Part model, mm, in its own coordinate system. Face numbers are marked on the shaded views. A direction names the side the tool comes from. Round coordinates to 2 decimals unless told otherwise and drop trailing zeros. Write each loop counter-clockwise with the first axis right and the second up, starting at its lowest first coordinate (ties: lowest second). Pieces come first, ordered by that corner, then holes.
```python
from build123d import *

# Parameters (mm, degrees)
SKETCH1_R                                    = 30
SKETCH1_R_2                                  = 20
BOSS_EXTRUDE1_DEPTH                          = 40
SKETCH2_W                                    = 2
SKETCH2_H                                    = 30
CUT_EXTRUDE1_DEPTH                           = 59.309518948
BOSS_EXTRUDE2_START                          = -40
BOSS_EXTRUDE2_DEPTH                          = 40
CBORE_FOR_M4_HEX_SOCKET_HEAD_CAP_SCR_2_COUNT = 2
CBORE_FOR_M4_HEX_SOCKET_HEAD_CAP_SCR_2_PITCH = 12
CBORE_FOR_M4_HEX_SOCKET_HEAD_CAP_SCR_3_COUNT = 2
CBORE_FOR_M4_HEX_SOCKET_HEAD_CAP_SCR_3_PITCH = 24
SKETCH6_R                                    = 3.75
CUT_EXTRUDE2_DEPTH                           = 66.946948375
F_5_4_5_4_DIAMETER_HOLE1_D                   = 4.2
SKETCH10_R                                   = 3
CUT_EXTRUDE3_DEPTH                           = 11
BOSS_EXTRUDE4_DEPTH                          = 20
BOSS_EXTRUDE4_DEPTH_BACK                     = 20
SKETCH13_R                                   = 17.5
SKETCH13_R_2                                 = 10
FILLET1_R                                    = 15


with BuildPart() as part:
    # Sketch1 → Boss-Extrude1 (new body)
    with BuildSketch(Plane(origin=(0, 0, 0), x_dir=(1, 0, 0), z_dir=(0, 1, 0))):
        with Locations(Location((0, 0, 0), (0, 0, 270))):
            Circle(SKETCH1_R)
        with Locations(Location((0, 0, 0), (0, 0, 270))):
            Circle(SKETCH1_R_2, mode=Mode.SUBTRACT)
    extrude(amount=BOSS_EXTRUDE1_DEPTH)

    # Sketch2 → Cut-Extrude1 (cut, through all)
    with BuildSketch(Plane(origin=(0, 40, 0), x_dir=(1, 0, 0), z_dir=(0, 1, 0))):
        with Locations((0, -15)):
            Rectangle(SKETCH2_W, SKETCH2_H)
    extrude(amount=-CUT_EXTRUDE1_DEPTH, mode=Mode.SUBTRACT)

    # Sketch3 → Boss-Extrude2 (add)
    with BuildSketch(Plane(origin=(0, 40, 0), x_dir=(1, 0, 0), z_dir=(0, 1, 0)).offset(BOSS_EXTRUDE2_START)):
        with BuildLine():
            Line((-1, -29.983328701), (-13, -29.983328701))
            Line((-13, -29.983328701), (-13, -27.037011669))
            ThreePointArc((-13, -27.037011669), (-7.153334608, -29.134683866), (-1, -29.983328701))
        make_face()
    extrude(amount=BOSS_EXTRUDE2_DEPTH)

    # Sketch5 → CBORE for M4 Hex Socket Head Cap Screw1 (revolve, cut)
    with BuildSketch(Plane(origin=(-13, 32, 24.979156528), x_dir=(0, 0, 1), z_dir=(0, 1, 0))):
        Polygon((0, 0), (0, 13.351936393), (2.25, 12), (2.25, 4), (3.75, 4), (3.75, 0), align=None)
    cbore_for_m4_hex_socket_head_cap_screw1 = revolve(axis=Axis((-19.35, 32, 24.979156528), (1, 0, 0)), mode=Mode.SUBTRACT)

    # CBORE for M4 Hex Socket Head Cap Scr 2: CBORE for M4 Hex Socket Head Cap Screw1 ×2
    with Locations(*[(0, -i * CBORE_FOR_M4_HEX_SOCKET_HEAD_CAP_SCR_2_PITCH, 0) for i in range(1, CBORE_FOR_M4_HEX_SOCKET_HEAD_CAP_SCR_2_COUNT)]):
        add(cbore_for_m4_hex_socket_head_cap_screw1, mode=Mode.SUBTRACT)

    # CBORE for M4 Hex Socket Head Cap Scr 3: CBORE for M4 Hex Socket Head Cap Screw1 ×2
    with Locations(*[(0, -i * CBORE_FOR_M4_HEX_SOCKET_HEAD_CAP_SCR_3_PITCH, 0) for i in range(1, CBORE_FOR_M4_HEX_SOCKET_HEAD_CAP_SCR_3_COUNT)]):
        add(cbore_for_m4_hex_socket_head_cap_screw1, mode=Mode.SUBTRACT)

    # Sketch6 → Cut-Extrude2 (cut, through all)
    with BuildSketch(Plane.ZY.offset(13)):
        with Locations((24.979156528, 32)):
            Circle(SKETCH6_R)
        with Locations((24.979156528, 20)):
            Circle(SKETCH6_R)
        with Locations((24.979156528, 8)):
            Circle(SKETCH6_R)
    extrude(amount=CUT_EXTRUDE2_DEPTH, mode=Mode.SUBTRACT)

    # Ø5.4 (5.4) Diameter Hole1 (through all)
    with Locations(Plane.ZY.offset(-1)):
        with Locations((24.979156528, 8), (24.979156528, 20), (24.979156528, 32)):
            Hole(F_5_4_5_4_DIAMETER_HOLE1_D / 2)

    # Sketch10 → Cut-Extrude3 (cut)
    with BuildSketch(Plane.ZY.offset(-22)):
        with Locations((24.979156528, 8)):
            Circle(SKETCH10_R)
        with Locations((24.979156528, 32)):
            Circle(SKETCH10_R)
        with Locations((24.979156528, 20)):
            Circle(SKETCH10_R)
    extrude(amount=CUT_EXTRUDE3_DEPTH, mode=Mode.SUBTRACT)

    # Sketch13 → Boss-Extrude4 (add, two sides: drawn at the far end of the back side and taken through both)
    # profile 1 of 3: a face of its own
    with BuildSketch(Plane(origin=(0, 0, 0), x_dir=(0, 0, -1), z_dir=(1, 0, 0)).offset(-BOSS_EXTRUDE4_DEPTH_BACK)):
        with BuildLine():
            ThreePointArc((28.5, 20), (33.625631329, 32.374368671), (46, 37.5))
            Line((46, 37.5), (30, 37.5))
            Line((30, 37.5), (28.5, 37.5))
            Line((28.5, 37.5), (28.5, 20))
        make_face()
    # profile 2 of 3: a face of its own
    with BuildSketch(Plane(origin=(0, 0, 0), x_dir=(0, 0, -1), z_dir=(1, 0, 0)).offset(-BOSS_EXTRUDE4_DEPTH_BACK)):
        with BuildLine():
            ThreePointArc((46, 2.5), (33.625631329, 7.625631329), (28.5, 20))
            Line((28.5, 20), (28.5, 2.5))
            Line((28.5, 2.5), (30, 2.5))
            Line((30, 2.5), (46, 2.5))
        make_face()
    # profile 3 of 3: a face of its own
    with BuildSketch(Plane(origin=(0, 0, 0), x_dir=(0, 0, -1), z_dir=(1, 0, 0)).offset(-BOSS_EXTRUDE4_DEPTH_BACK)):
        with Locations((46, 20)):
            Circle(SKETCH13_R)
        with Locations((46, 20)):
            Circle(SKETCH13_R_2, mode=Mode.SUBTRACT)
    extrude(amount=BOSS_EXTRUDE4_DEPTH + BOSS_EXTRUDE4_DEPTH_BACK)

    # Fillet1
    # the kernel refuses this fillet: 15 mm, written as the material it adds along each edge
    with BuildSketch(Plane(origin=(9.367496998, 37.5, -28.5), x_dir=(0.8228917781054501, 0, 0.5681981357998729), z_dir=(0, -1, 0))) as fillet1_piece_1:
        with BuildLine():
            CenterArc((21.213026524, -14.387505004), FILLET1_R, 106.429799285, 39.762375137)
            Line((8.749399301, -6.041368385), (0, 0))
            ThreePointArc((0, 0), (8.48521061, -1.224989993), (16.970421219, 0))
        make_face()
    extrude(amount=35)
    with BuildSketch(Plane(origin=(-9.367496998, 37.5, -28.5), x_dir=(-0.8228917781054502, 0, 0.5681981357998726), z_dir=(0, -1, 0))) as fillet1_piece_2:
        with BuildLine():
            CenterArc((21.213026524, 14.387505004), FILLET1_R, 213.807825578, 39.762375137)
            Line((8.749399301, 6.041368385), (0, 0))
            ThreePointArc((0, 0), (8.48521061, 1.224989993), (16.970421219, 0))
        make_face()
    extrude(amount=35)


solid = part.part
```
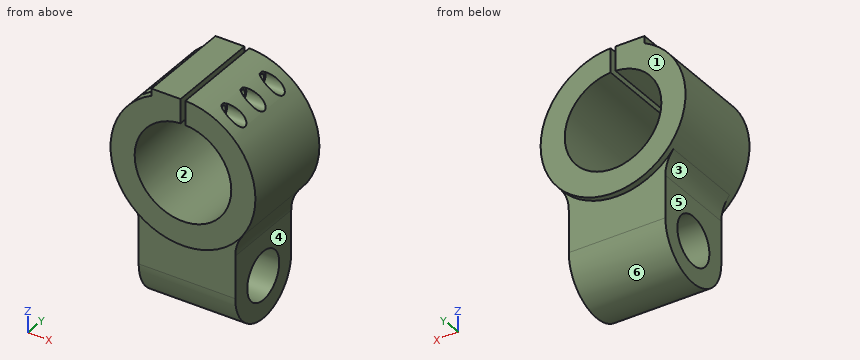
Q1. Cut at D-D on y = 26.5. Write the cut outline in (x, z), plus the area to 3 significant figures.
Values follow:
outline: (-23.33, -18.86) arc R15 cw to (-20, -28.5) - (-20, -38.4) - (20, -38.4) - (20, -28.5) arc R15 cw to (23.33, -18.86) arc R30 ccw to (1, 29.98) - (1, 19.97) arc R20 cw (long way) to (-1, 19.97) - (-1, 29.98) - (-13, 29.98) - (-13, 27.04) arc R30 ccw to start; (-20, -62.25) - (20, -62.25) - (20, -53.6) - (-20, -53.6) - close
area: 2,350 mm2
Q2. Cut at A-A on z = 0. Write the cut outline in (x, y), plus the area to 3 significant figures.
Values follow:
outline: (-30, 0) - (-20, 0) - (-20, 40) - (-30, 40) - close; (20, 0) - (30, 0) - (30, 40) - (20, 40) - close
area: 800 mm2
Q3. Mould opens along X. For the marked faces 1, 2 and 3 say: +X half, -X half, draft (parallel to the pull), parting line (faces both ways), or undercut.
Values follow:
face 1: draft
face 2: undercut
face 3: -X half
Q4. Drop flat-ended pins along their axis: pin 1 (5.5 mm diameter, centred on y = 32, z = 24.98, fed in from -X); pin 2 (8 mm diameter, centred on y = 21.5, z = 23, fed in from -X); pin 3 (1.5 mm diameter, centred on y = 24.5, z = -29.5, fed in from -X); pin 4 (8 mm diameter, centred on x = 9, z = -30.5, fed in from +Y). Give the stop position or say it passes through.
Values follow:
pin 1: stops at x = -9
pin 2: stops at x = -23.22
pin 3: stops at x = -20
pin 4: stops at y = 40
Q5. Wall check: L1, parallel to Z at x = 14.5, y = 12; L2, parallel to Z at x = 16, y = 20.5; L3, parallel to Y at x = -9.5, z = -46. Give the ranges that are in metal, low to high.
Values follow:
L1: z = -61.56 to -52, -40 to -13.77, 13.77 to 26.26
L2: z = -63.49 to -55.99, -36.01 to -12, 12 to 22.02
L3: y = 2.5 to 10, 30 to 37.5
Q6. Cut at B-B on x = 3.5. Write the cut outline in (y, z).
Values follow:
outline: (0, -29.8) - (2.5, -29.8) - (2.5, -46) arc R17.5 ccw to (37.5, -46) - (37.5, -29.8) - (40, -29.8) - (40, -19.69) - (0, -19.69) - close; (0, 19.69) - (40, 19.69) - (40, 29.8) - (0, 29.8) - close; hole circle Ø4.2 at (8, 24.98); hole circle Ø20 at (20, -46); hole circle Ø4.2 at (20, 24.98); hole circle Ø4.2 at (32, 24.98)
Q7. Cut at C-C on x = -19. Write the cut outline in (y, z) (3 decimals), plus the area to 3 significant figures.
Values follow:
outline: (0, -23.216) - (2.5, -23.216) - (2.5, -46) arc R17.5 ccw to (37.5, -46) - (37.5, -23.216) - (40, -23.216) - (40, -6.245) - (0, -6.245) - close; (0, 6.245) - (40, 6.245) - (40, 23.216) - (35.31, 23.216) arc R3.75 cw to (28.69, 23.216) - (23.31, 23.216) arc R3.75 cw to (16.69, 23.216) - (11.31, 23.216) arc R3.75 cw to (4.69, 23.216) - (0, 23.216) - close; hole circle Ø20 at (20, -46)
area: 2,290 mm2
Q8. Which spindle directions (+Z, -Z, +X, -X, +Y, -Y) get a long thin tool onto all of the face, cutting with end or side? Do the marked faces 4, 5 and 6. Say none if no direction does.
Values follow:
face 4: -Z, +X, +Y, -Y
face 5: -Z, -X, +Y, -Y
face 6: -Z, +X, -X
